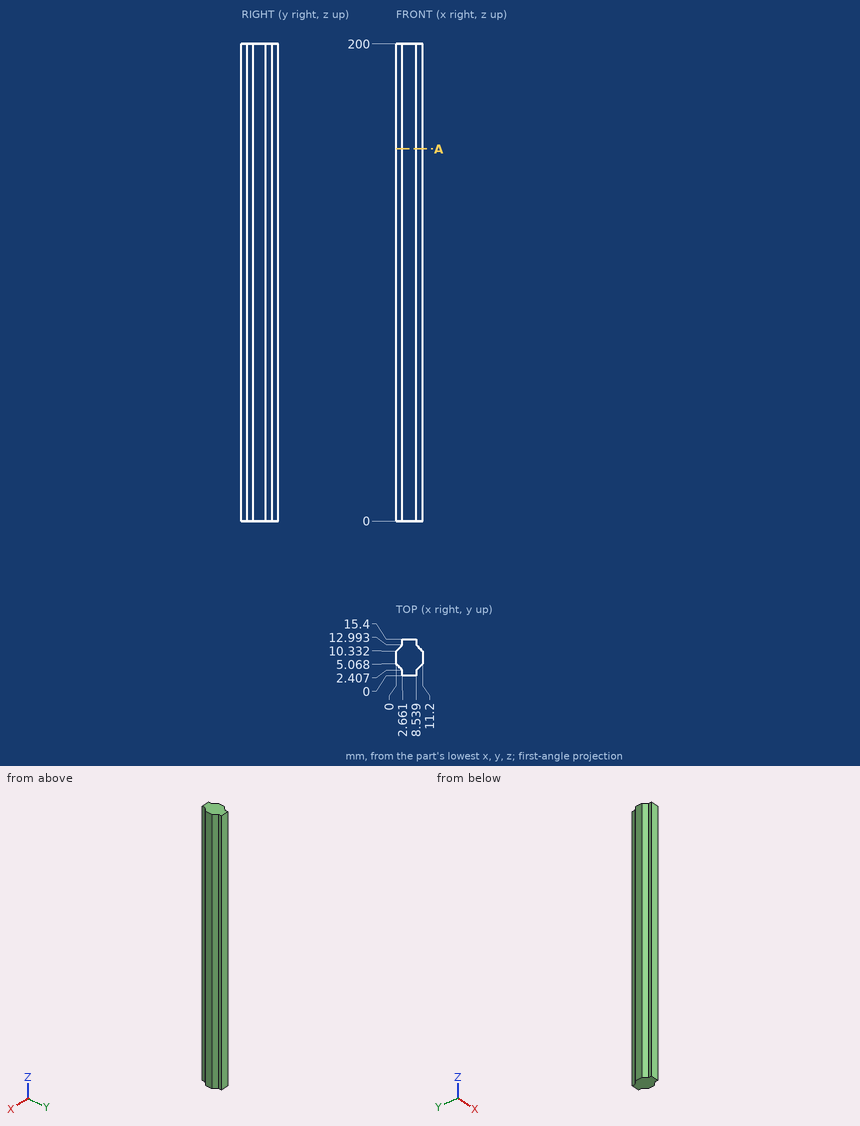
Part print with two shaded views. Sizes in mm from the minimum x, y, z corner. Give positions to 0.01 mm unless a question says otherwise; leave off trailing zeros. Write each loop counter-clockwise with the first axis right and the second up, starting at its lowest first coordinate (ties: lowest second). Pieces come first, ordered by that corner, then holes.
1) Cut at A-A on z = 156. Write the cut outline in (x, y).
Resolved:
outline: (0, 5.07) - (2.66, 2.41) - (2.66, 0) - (8.54, 0) - (8.54, 2.41) - (11.2, 5.07) - (11.2, 10.33) - (8.54, 12.99) - (8.54, 15.4) - (2.66, 15.4) - (2.66, 12.99) - (0, 10.33) - close
2) Probe L1, parallel to Y at x = 9, z = 39; L2, parallel to Y at x = 9.5, z = 56.5; L3, parallel to X at y = 1, z = 124. List the from-to ranges inside material, lowest first.
Resolved:
L1: y = 2.87 to 12.53
L2: y = 3.37 to 12.03
L3: x = 2.66 to 8.54
3) Pin check, flat tips, straight feed: pin 1 (1.9 mm diameter, centred on y = 14.5, z = 99, fed in from +X); pin 2 (1.2 mm diameter, centred on y = 1, z = 148, fed in from -X). Stop position of each tip, or through.
Resolved:
pin 1: stops at x = 8.54
pin 2: stops at x = 2.66
